Here's the drawing with two shaded views (mm, measured from the low corner). I have some questions. A direction names the side the tool comes from. Give positions to 0.01 mm unless a question says otherwise; leave off trailing zeros. Write each loop counter-clockwise with the first axis right and the second up, starting at its lowest first coordinate (ties: lowest second). Pieces come first, ordered by that corner, then holes. Notation, with made-up numbers: (-20, 28.5) -> (14, 28.5) arc R29 ccw to (14, 51.5) -> close; hole circle Ø2 at (59.25, 16). An arc over 180 degrees is marked (long way). One line per question, with ' | ' between items.
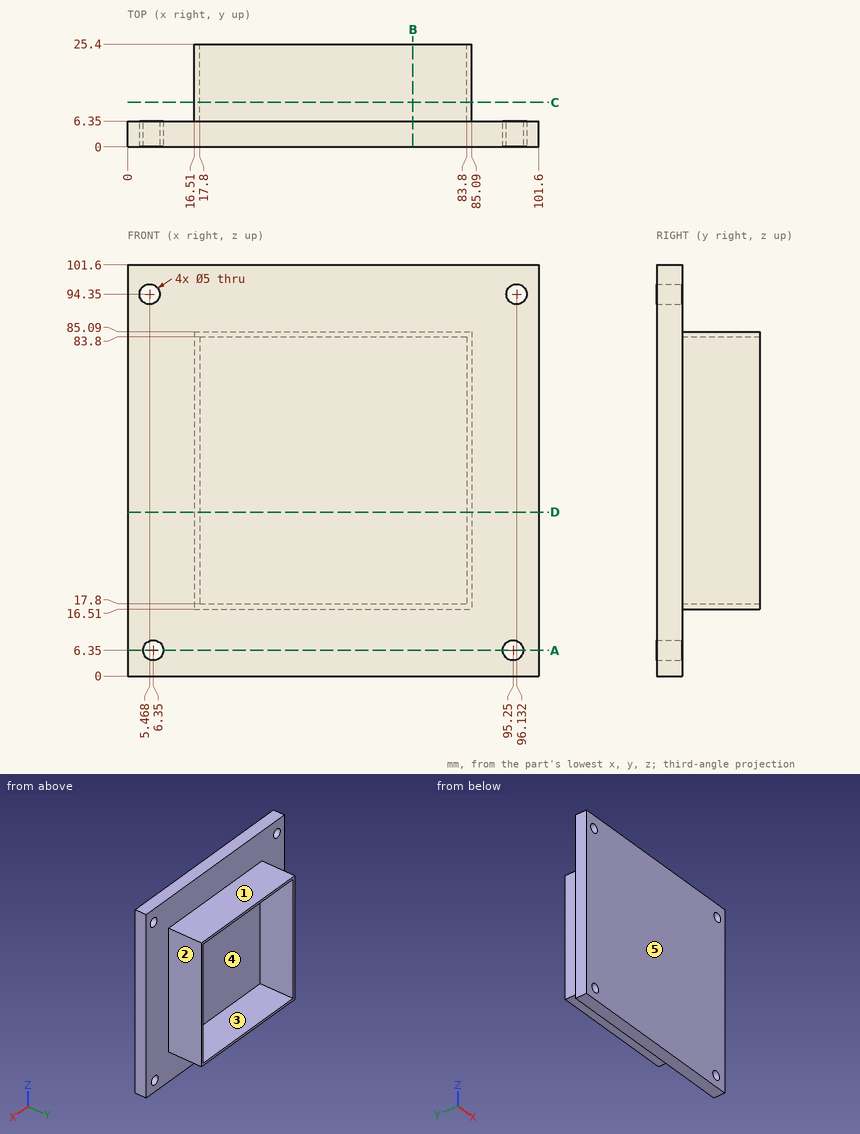
Q1. If we mould it in two halves opening along X, with no side actions, what happens to the marked faces 1, 2 and 3? For each: +X half, -X half, draft (parallel to the pull), parting line (faces both ways), or undercut.
Answer below:
face 1: draft | face 2: +X half | face 3: undercut
Q2. Imagine slicing it at C-C on y = 11. Please give me the cut outline in (x, z).
Answer below:
outline: (16.51, 16.51) -> (85.09, 16.51) -> (85.09, 85.09) -> (16.51, 85.09) -> close; hole (17.8, 17.8) -> (83.8, 17.8) -> (83.8, 83.8) -> (17.8, 83.8) -> close
Q3. Will these pins go through, and if not, where does the flat tip stop? pin 1 (4 mm diameter, centred on y = 19, z = 74.5, fed in from -X); pin 2 (8 mm diameter, centred on x = 49.5, y = 14, fed in from +Z); pin 3 (15 mm diameter, centred on y = 17, z = 34, fed in from +X).
Answer below:
pin 1: stops at x = 16.51 | pin 2: stops at z = 85.09 | pin 3: stops at x = 85.09
Q4. If I drill on line 1 along X through (y, z) = (4, 6.35); line 2 along X through (y, z) = (17, 72), over which ranges is the centre line in solid material (lowest first)?
Answer below:
line 1: x = 0 to 3.85, 8.85 to 92.75, 97.75 to 101.6 | line 2: x = 16.51 to 17.8, 83.8 to 85.09
Q5. Imagine slicing it at D-D on z = 40.5. Please give me the cut outline in (x, y).
Answer below:
outline: (0, 0) -> (101.6, 0) -> (101.6, 6.35) -> (85.09, 6.35) -> (85.09, 25.4) -> (83.8, 25.4) -> (83.8, 6.35) -> (17.8, 6.35) -> (17.8, 25.4) -> (16.51, 25.4) -> (16.51, 6.35) -> (0, 6.35) -> close
Q6. Imagine slicing it at A-A on z = 6.35. Please give me the cut outline in (x, y).
Answer below:
outline: (0, 0) -> (3.85, 0) -> (3.85, 6.35) -> (0, 6.35) -> close; (8.85, 0) -> (92.75, 0) -> (92.75, 6.35) -> (8.85, 6.35) -> close; (97.75, 0) -> (101.6, 0) -> (101.6, 6.35) -> (97.75, 6.35) -> close
Q7. Imagine slicing it at B-B on x = 70.5. Please give me the cut outline in (y, z).
Answer below:
outline: (0, 0) -> (6.35, 0) -> (6.35, 16.51) -> (25.4, 16.51) -> (25.4, 17.8) -> (6.35, 17.8) -> (6.35, 83.8) -> (25.4, 83.8) -> (25.4, 85.09) -> (6.35, 85.09) -> (6.35, 101.6) -> (0, 101.6) -> close
Q8. On a 3-axis mill with a long thin cutter (end or side, diameter ignored), from which of +Z, -Z, +X, -X, +Y, -Y can I reach the whole of each face in a straight line? I mean the marked faces 4 and 5. Say none if no direction works.
Answer below:
face 4: +Y | face 5: +Z, -Z, +X, -X, -Y
